The listing builds one solid part. Answer for the finished solid, in the listing's coordinates (mm). A direction names the side the tool comes from. Give positions to 0.01 mm unless a question says otherwise; leave off trailing zeros. Write each loop counter-clockwise with the first axis right and the second up, starting at its lowest first coordinate (ties: lowest second). Pieces come first, ordered by that corner, then holes. Notation, with made-up numbers: (63.5, 3.5) -> (83.5, 3.5) arc R20 ccw to (83.5, 10.5) -> close; hole circle Ø4 at (-20, 32.25). An arc over 180 degrees is marked (long way). Put each result on its own line as item: value. Start each with the question number.
1) A cutting plane is placed at D-D (y = -17.5). Write down the section's boundary in (x, z).
2) For a pull along X with two mould halves and no side action, classify faces 4 (the flat face through (52, -110, 19)), 5 (the cylindrical face through (-34.685, -14.79, -156.195)), 6 (the flat face through (11, -40, -24)) as released by +X, released by -X, zero draft, split by the parting line, or undercut.
3) For faces 1 (the cylindrical face through (23.846, -1.975, 7.509)), 2 (the flat face through (33, 0, -33)), 3 (the cylindrical face through (-11.923, -75.49, -53.692)), determine the directions among +Z, -Z, +X, -X, +Y, -Y from which every point of the face is accessible in a straight line to the end or side of a thin tool.
4) Flat-ended cylindrical pins translate along their axes: pin 1 Ø10 at (y, z) = (-22, 85) entering from +X; pin 2 Ø12 at (x, y) = (90, -48.5) entering from +Z; pin 3 Ø8.5 at (x, z) = (-85, 0) entering from +Y. Find the tip coordinate at first contact, or state that the pin passes through.
5) Find the intervals of material crossed by line 1 along Z through (x, y) = (85, -21.25); line 2 along X through (y, z) = (-46, 7.5); line 3 along X through (y, z) = (-54, -8.5), in increasing order. Write a range as from..to.
6) A cutting plane is placed at B-B (x = 0). Write down the section's boundary in (y, z), then the cut area to 3 significant figures.
7) A cutting plane is placed at C-C (y = 24). Write down the section's boundary in (x, z), then the cut area to 3 significant figures.
8) A cutting plane is placed at A-A (z = 0). Write down the section's boundary in (x, y), then the cut area to 3 significant figures.
from build123d import *

# Parameters (mm, degrees)
F0_R     = 160
F0_R_2   = 50
F0_R_3   = 42.35
F0_R_4   = 25
F1_DEPTH = 110
F2_DEPTH = 35
F3_SIZE  = 80
F4_R     = 55
F5_DEPTH = 70
F6_R     = 7
F7_DEPTH = 30


with BuildPart() as f1:
    # F0 (on Front) → F1 (new body)
    with BuildSketch(Plane.XZ):
        Circle(F0_R)
        Circle(F0_R_2, mode=Mode.SUBTRACT)
        Circle(F0_R_2)
        Circle(F0_R_3, mode=Mode.SUBTRACT)
        Circle(F0_R_3)
        Circle(F0_R_4, mode=Mode.SUBTRACT)
    extrude(amount=F1_DEPTH)

    # F0 (on Front) → F2 (join)
    with BuildSketch(Plane.XZ):
        Circle(F0_R_3)
        Circle(F0_R_4, mode=Mode.SUBTRACT)
    extrude(amount=-F2_DEPTH)

    # F3
    f3_edges = [f1.edges().sort_by_distance(p)[0] for p in [
        (-160, -110, 0),
    ]]
    chamfer(f3_edges, length=F3_SIZE)

    # F4 (on face) → F5 (cut)
    with BuildSketch(Plane.XZ.offset(110)):
        Circle(F4_R)
    extrude(amount=-F5_DEPTH, mode=Mode.SUBTRACT)

    # F6 (on face) → F7 (cut)
    with BuildSketch(Plane(origin=(0, 0, 0), x_dir=(-1, 0, 0), z_dir=(0, 1, 0))):
        with Locations((-85, 0)):
            Circle(F6_R)
        with Locations((85, 0)):
            Circle(F6_R)
    extrude(amount=-F7_DEPTH, mode=Mode.SUBTRACT)


solid = f1.part
Reply:
1. outline: circle Ø320 at (0, 0); hole circle Ø14 at (-85, 0); hole circle Ø50 at (0, 0); hole circle Ø14 at (85, 0)
2. face 4: zero draft
2. face 5: split by the parting line
2. face 6: undercut
3. face 1: +Y, -Y
3. face 2: +Y
3. face 3: -Y
4. pin 1: stops at x = 138.56
4. pin 2: stops at z = 118.11
4. pin 3: stops at y = -30
5. line 1: z = -135.55..-7, 7..135.55
5. line 2: x = -143.8..-54.49, 54.49..143.8
5. line 3: x = -135.73..-54.34, 54.34..135.73
6. outline: (-110, -80) -> (-30, -160) -> (0, -160) -> (0, -42.35) -> (35, -42.35) -> (35, -25) -> (-40, -25) -> (-40, -55) -> (-110, -55) -> close; (-110, 55) -> (-40, 55) -> (-40, 25) -> (35, 25) -> (35, 42.35) -> (0, 42.35) -> (0, 160) -> (-30, 160) -> (-110, 80) -> close
6. area: 20,300 mm2
7. outline: circle Ø84.7 at (0, 0); hole circle Ø50 at (0, 0)
7. area: 3,670 mm2
8. outline: (-160, -30) -> (-80, -110) -> (-55, -110) -> (-55, -40) -> (-25, -40) -> (-25, 35) -> (-42.35, 35) -> (-42.35, 0) -> (-78, 0) -> (-78, -30) -> (-92, -30) -> (-92, 0) -> (-160, 0) -> close; (25, -40) -> (55, -40) -> (55, -110) -> (80, -110) -> (160, -30) -> (160, 0) -> (92, 0) -> (92, -30) -> (78, -30) -> (78, 0) -> (42.35, 0) -> (42.35, 35) -> (25, 35) -> close
8. area: 19,500 mm2
